Check sheet for the drawn part. Datum: minimum x, y, z corner. Units: mm. A direction names the side the tool comes from. Coordinates: 2 decimals unless noted, no trailing zeros. Order: outer loops, then holes, each group sorted by start corner. A loop starts at its lowest first (then second) coordinate and runs counter-clockwise, first axis right, second up. Notation, with made-up numbers: (-13, -40) - (23, -40) arc R21 ccw to (23, -2) - close; hole circle Ø1 at (57, 18.25). An arc over 180 degrees is marked (long way). Return JSON: item names as keys, results as strings. Group by question number.
Item 1: Section check B-B on y = 78.5. Enter the section's corners in (x, z).
Item 2: Section check C-C on x = 248. Enter the section's corners in (y, z).
Item 3: Draft check along X on the marked faces 3, 4 and 5. Enter one of: pulls with the +X half, pulls with the -X half, needs draft (parallel to the pull), parting line crosses it, or undercut.
Item 4: Section check A-A on z = 90. Enter the section's corners in (x, y).
Item 5: Gauge pin test, flat end, axial feed: pin 1 (10 mm diameter, centred on x = 385.5, y = 57, fed in from +Z). Record the tip position at first contact, or that the pin passes through.
Item 6: Tool access check on the marked faces 1 and 2. Record the directions out of +Z, -Z, +X, -X, +Y, -Y that give a thin tool (end or side, any length) a straight path to the whole face; none if there is none.
Item 7: Scan lines: probe 1 along Y at (x, z) = (109, 77); probe 2 along X at (y, z) = (474.5, 82); probe 3 along Z at (x, y) = (163, 444). Record each from-to range of solid material in increasing order.
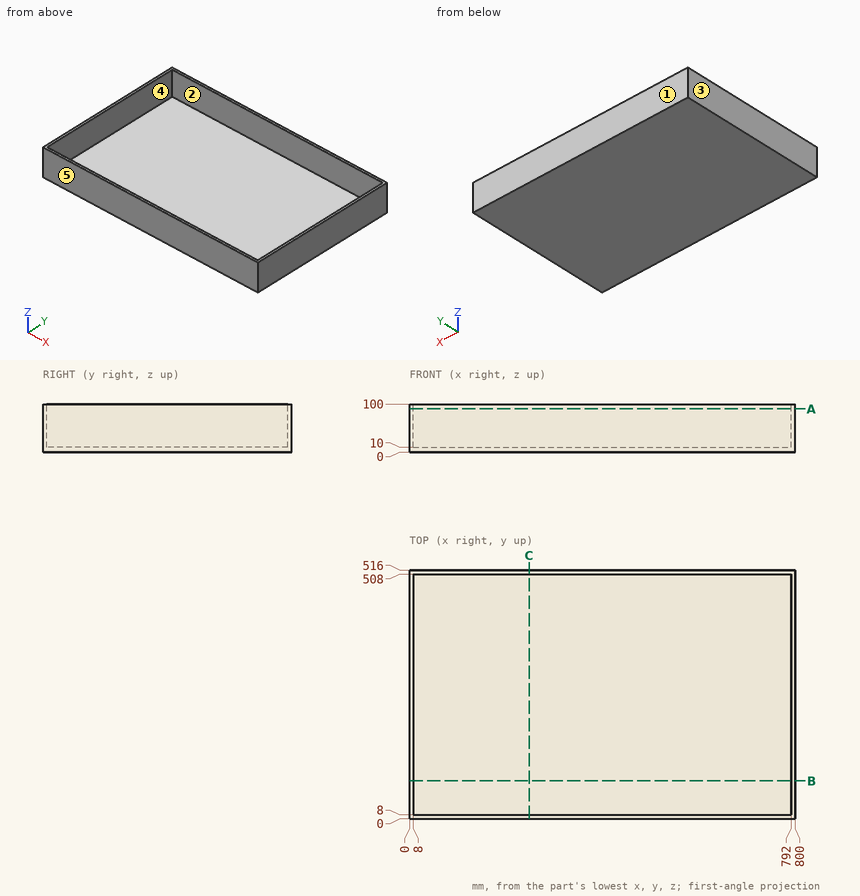
Computed:
{
 "1": {"outline": "(0, 0) - (800, 0) - (800, 100) - (792, 100) - (792, 10) - (8, 10) - (8, 100) - (0, 100) - close"},
 "2": {"outline": "(0, 0) - (516, 0) - (516, 100) - (508, 100) - (508, 10) - (8, 10) - (8, 100) - (0, 100) - close"},
 "3": {"face 3": "pulls with the -X half", "face 4": "undercut", "face 5": "needs draft"},
 "4": {"outline": "(0, 0) - (800, 0) - (800, 516) - (0, 516) - close; hole (8, 8) - (792, 8) - (792, 508) - (8, 508) - close"},
 "5": {"pin 1": "stops at z = 10"},
 "6": {"face 1": "+Z, -Z, +X, -X, +Y", "face 2": "+Z"},
 "7": {"probe 1": "y = 0 to 8, 508 to 516", "probe 2": "x = 0 to 8, 792 to 800", "probe 3": "z = 0 to 10"}
}
